from build123d import *


with BuildPart() as part:
    # Esquisse1 → Révolution1 (revolve)
    with BuildSketch(Plane.XZ, mode=Mode.PRIVATE) as r_volution1_sk:
        Polygon((17.5, 62), (0, 51.484939167), (0, 0), (29, 0), (30, 1), (30, 69), (29, 70), (17.5, 70), align=None)
    revolve(r_volution1_sk.sketch.rotate(Axis((0, 0, 70), (0, 0, -1)), 180), axis=Axis((0, 0, 70), (0, 0, -1)))


solid = part.part
CAD build for the part. Positions are in the model's coordinates, mm. A direction names the side the tool comes from. Coordinates: 2 decimals unless noted, no trailing zeros. Order: outer loops, then holes, each group sorted by start corner. A loop starts at its lowest first (then second) coordinate and runs counter-clockwise, first axis right, second up.
Item 1: Pin check, flat tips, straight feed: pin 1 Ø3 at (y, z) = (12.5, 40.5) entering from -X; pin 2 Ø1.5 at (x, z) = (10.5, 18) entering from -Y; pin 3 Ø5 at (x, z) = (-20.5, 46.5) entering from -Y. Stop position of each tip, or through.
Check sheet entries:
pin 1: stops at x = -27.91
pin 2: stops at y = -28.37
pin 3: stops at y = -24
Item 2: Drill centre lines: L1, parallel to Y at x = 0, z = 66; L2, parallel to X at y = -10, z = 11.5; L3, parallel to Y at x = -26, z = 23.5. Where is each one in solid material? Low to high.
Check sheet entries:
L1: y = -30 to -17.5, 17.5 to 30
L2: x = -28.28 to 28.28
L3: y = -14.97 to 14.97
Item 3: Band-saw the part on B-B on z = 10.5. List the corners of the cut face in (x, y), plus the area to 3 significant figures.
Check sheet entries:
outline: circle Ø60 at (0, 0)
area: 2,830 mm2
Item 4: Two-plate mould, pull along Y, no slides. Class faces 1 (the face through (-12.5, -12.5, 70)), 2 (the face through (-16.128, 25.296, 35.476)), 3 (the face through (0.606, -2.728, 53.164)): +Y half, -Y half, draft (parallel to the pull), parting line (faces both ways), or undercut.
Check sheet entries:
face 1: draft
face 2: parting line
face 3: undercut
Item 5: 3-axis set-ups, long thin cutter, end or side, ignore diameter. For faces 4 (the face through (3.794, -17.084, 65.944)), 5 (the face through (0, 0, 0)): which of +Z, -Z, +X, -X, +Y, -Y reach the whole face in a straight line?
Check sheet entries:
face 4: +Z
face 5: -Z, +X, -X, +Y, -Y
Item 6: Band-saw the part on A-A on z = 65. List the corners of the cut face in (x, y).
Check sheet entries:
outline: circle Ø60 at (0, 0); hole circle Ø35 at (0, 0)
